Here's the drawing with two shaded views (mm, measured from the low corner). I have some questions. Give positions to 0.01 mm unless a question says otherwise; leave off trailing zeros. Order: outer loops, then holes, each group sorted by start corner. A loop starts at its lowest first (then second) coordinate and runs counter-clockwise, first axis right, second up. Notation, with made-up numbers: M -12.5,79.5 L -5.5,79.5 A10 ccw -5.5,87.5 Z; hole C 34.25,-1.75 d4. An arc over 180 degrees is marked long. Write each question's results on one line, items separated by ' | '.
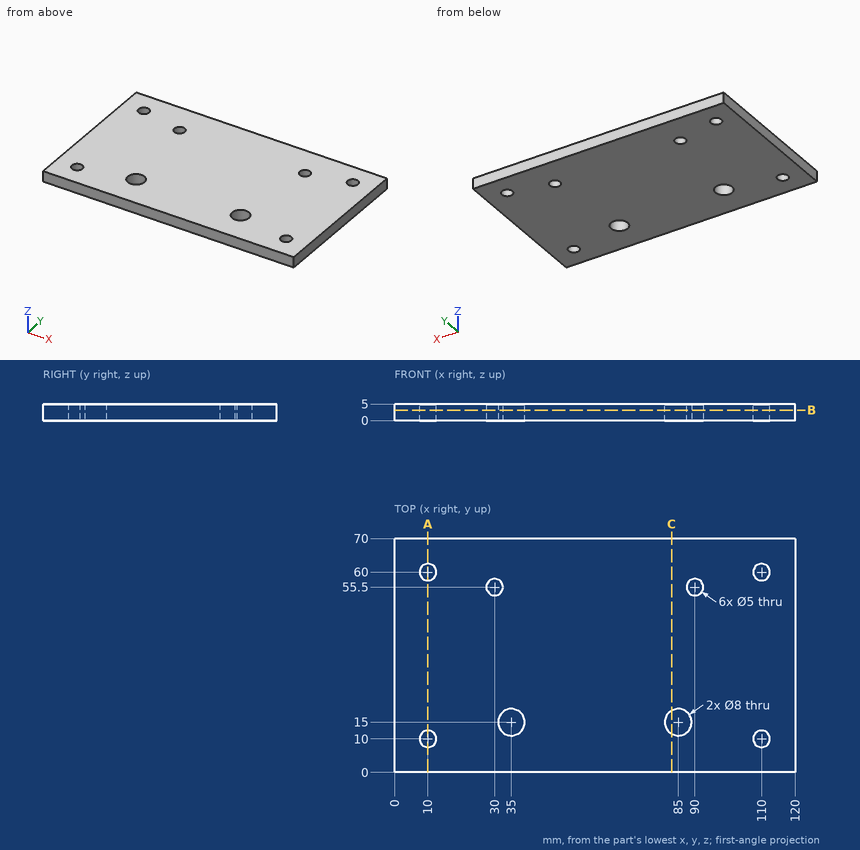
(1) I need wall thicknesses on L1, parallel to Y at x = 110, z = 1; L2, parallel to Y at x = 30, z = 1.1; L3, parallel to Y at x = 8, z = 1.05. Which ranges of each line are inside material? Lowest first, please. Write a range as from..to.
Data:
L1: y = 0..7.5, 12.5..57.5, 62.5..70 | L2: y = 0..53, 58..70 | L3: y = 0..8.5, 11.5..58.5, 61.5..70
(2) Imagine slicing it at C-C, the plane x = 83. Write out the boundary of the cut face in (y, z), plus the area to 3 significant figures.
Data:
outline: M 0,0 L 11.54,0 L 11.54,5 L 0,5 Z; M 18.46,0 L 70,0 L 70,5 L 18.46,5 Z | area: 315 mm2
(3) Imagine slicing it at B-B, the plane z = 3.15. Count the separate pieces of the cut face and the enclosed holes in it, plus the area to 3 significant figures.
Data:
separate pieces: 1 | enclosed holes: 8 | area: 8,180 mm2
(4) Will this pin go through, and if not, where does the flat tip stop? P1, Ø4.5, axis at x = 10, y = 60, coming from the +Z side.
Data:
P1: passes through
(5) Imagine slicing it at A-A, the plane x = 10. Write out the boundary of the cut face in (y, z).
Data:
outline: M 0,0 L 7.5,0 L 7.5,5 L 0,5 Z; M 12.5,0 L 57.5,0 L 57.5,5 L 12.5,5 Z; M 62.5,0 L 70,0 L 70,5 L 62.5,5 Z
